Source: CAD feature listing. Evaluate the final solid. Frame: model axes, mm. Face numbers are marked on the shaded views. A direction names the side the tool comes from. Give positions to 0.01 mm unless a question says otherwise; leave off trailing zeros. Write each loop counter-clockwise with the first axis right and the second up, starting at its lowest first coordinate (ties: lowest second). Pieces come first, ordered by that corner, then holes. Notation, with made-up numbers: (-7.75, 63) -> (24.25, 63) arc R15 ccw to (24.25, 72) -> close; hole circle Ø1 at (75.25, 72). An arc over 180 degrees is marked (long way). Write item = value, one per line.
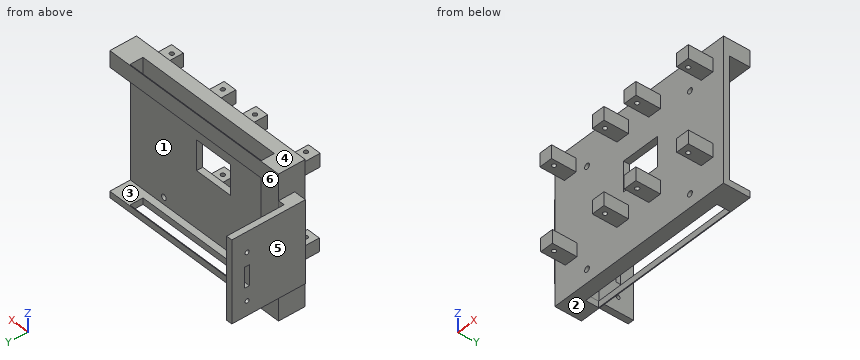
from build123d import *

# Parameters (mm, degrees)
SKETCH_1_W           = 95
SKETCH_1_H           = 70
SKETCH_1_R           = 1.35
SKETCH_1_W_2         = 19.026786566
SKETCH_1_H_2         = 14.673074928
EXTRUDE_1_DEPTH      = 13
SKETCH_3_W           = 85
SKETCH_3_H           = 59
CUT_EXTRUDE_1_DEPTH  = 10
SKETCH_4_W           = 6.551363844
SKETCH_4_H           = 6.551363844
EXTRUDE_2_DEPTH      = 12
SKETCH_7_W           = 6.551363844
SKETCH_7_H           = 6.551363844
EXTRUDE_3_DEPTH      = 12
SKETCH_9_R           = 1
CUT_EXTRUDE_4_DEPTH  = 63
SKETCH_5_R           = 1
CUT_EXTRUDE_5_DEPTH  = 56
SKETCH_12_W          = 6.551363844
SKETCH_12_H          = 6.551363844
EXTRUDE_4_DEPTH      = 12
SKETCH_13_R          = 1
CUT_EXTRUDE_6_DEPTH  = 9
SKETCH_15_R          = 1
CUT_EXTRUDE_7_DEPTH  = 51
SKETCH_17_W          = 6.551363844
SKETCH_17_H          = 6.551363844
EXTRUDE_5_DEPTH      = 12
SKETCH_18_R          = 1
CUT_EXTRUDE_8_DEPTH  = 12
SKETCH_19_R          = 1
CUT_EXTRUDE_9_DEPTH  = 12
SKETCH_20_W          = 40
SKETCH_20_H          = 7.86503053
EXTRUDE_6_DEPTH      = 6
SKETCH_21_W          = 2.903775518
SKETCH_21_H          = 40
EXTRUDE_7_DEPTH      = 28
SKETCH_22_W          = 74
SKETCH_22_H          = 6.331212291
CUT_EXTRUDE_10_DEPTH = 78
SKETCH_23_W          = 10
SKETCH_23_H          = 2.4
CUT_EXTRUDE_13_DEPTH = 10
SKETCH_25_R          = 1
CUT_EXTRUDE_14_DEPTH = 10


with BuildPart() as part:
    # 草图1 → 凸台-拉伸1 (new body)
    with BuildSketch(Plane(origin=(0, 0, 0), x_dir=(1, 0, 0), z_dir=(0, 1, 0))):
        with Locations((21.0257099, -17.142747506)):
            Rectangle(SKETCH_1_W, SKETCH_1_H)
        with Locations((49.670533911, 11.329362359)):
            Circle(SKETCH_1_R, mode=Mode.SUBTRACT)
        with Locations((49.670533911, -37.670637641)):
            Circle(SKETCH_1_R, mode=Mode.SUBTRACT)
        with Locations((-8.329466089, -37.670637641)):
            Circle(SKETCH_1_R, mode=Mode.SUBTRACT)
        with Locations((-8.329466089, 11.329362359)):
            Circle(SKETCH_1_R, mode=Mode.SUBTRACT)
        with Locations((21.72534394, -20.076013692)):
            Rectangle(SKETCH_1_W_2, SKETCH_1_H_2, mode=Mode.SUBTRACT)
    extrude(amount=EXTRUDE_1_DEPTH)

    # 草图3 → 切除-拉伸1 (cut)
    with BuildSketch(Plane(origin=(0, 13, 0), x_dir=(1, 0, 0), z_dir=(0, 1, 0))):
        with Locations((26.0257099, -14.722914633)):
            Rectangle(SKETCH_3_W, SKETCH_3_H)
    extrude(amount=-CUT_EXTRUDE_1_DEPTH, mode=Mode.SUBTRACT)

    # 草图4 → 凸台-拉伸2 (add)
    with BuildSketch(Plane.XZ):
        with Locations((-17.262018052, 1.397045451)):
            Rectangle(SKETCH_4_W, SKETCH_4_H)
        with Locations((-17.755298179, 42.036450596)):
            Rectangle(SKETCH_4_W, SKETCH_4_H)
        with Locations((59.313437853, 1.397045451)):
            Rectangle(SKETCH_4_W, SKETCH_4_H)
        with Locations((59.313437853, 42.036450596)):
            Rectangle(SKETCH_4_W, SKETCH_4_H)
    extrude(amount=EXTRUDE_2_DEPTH)

    # 草图7 → 凸台-拉伸3 (add)
    with BuildSketch(Plane.XZ):
        with Locations((29.762074009, 2.155967477)):
            Rectangle(SKETCH_7_W, SKETCH_7_H)
    extrude(amount=EXTRUDE_3_DEPTH)

    # 草图9 → 切除-拉伸4 (cut)
    with BuildSketch(Plane(origin=(0, 0, -1.119714445), x_dir=(-1, 0, 0), z_dir=(0, 0, -1))):
        with Locations((-29.819487591, -8.583293227)):
            Circle(SKETCH_9_R)
    extrude(amount=-CUT_EXTRUDE_4_DEPTH, mode=Mode.SUBTRACT)

    # 草图5 → 切除-拉伸5 (cut)
    with BuildSketch(Plane(origin=(0, 0, -1.878636471), x_dir=(-1, 0, 0), z_dir=(0, 0, -1))):
        with Locations((-58.566110561, -8.583293227)):
            Circle(SKETCH_5_R)
    extrude(amount=-CUT_EXTRUDE_5_DEPTH, mode=Mode.SUBTRACT)

    # 草图12 → 凸台-拉伸4 (add)
    with BuildSketch(Plane(origin=(0, 0, 0), x_dir=(-1, 0, 0), z_dir=(0, -1, 0))):
        with Locations((-29.762074009, -42.795372621)):
            Rectangle(SKETCH_12_W, SKETCH_12_H)
    extrude(amount=EXTRUDE_4_DEPTH)

    # 草图13 → 切除-拉伸6 (cut)
    with BuildSketch(Plane.XY.offset(46.071054543)):
        with Locations((29.819487591, -8.583293227)):
            Circle(SKETCH_13_R)
    extrude(amount=-CUT_EXTRUDE_6_DEPTH, mode=Mode.SUBTRACT)

    # 草图15 → 切除-拉伸7 (cut)
    with BuildSketch(Plane.XY.offset(45.312132518)):
        with Locations((-17.007970887, -8.583602404)):
            Circle(SKETCH_15_R)
    extrude(amount=-CUT_EXTRUDE_7_DEPTH, mode=Mode.SUBTRACT)

    # 草图17 → 凸台-拉伸5 (add)
    with BuildSketch(Plane(origin=(0, 0, 0), x_dir=(-1, 0, 0), z_dir=(0, -1, 0))):
        with Locations((-11.796065665, -42.036450596)):
            Rectangle(SKETCH_17_W, SKETCH_17_H)
        with Locations((-11.796065665, -1.397045451)):
            Rectangle(SKETCH_17_W, SKETCH_17_H)
    extrude(amount=EXTRUDE_5_DEPTH)

    # 草图18 → 切除-拉伸8 (cut)
    with BuildSketch(Plane.XY.offset(45.312132518)):
        with Locations((11.738652082, -8.583602404)):
            Circle(SKETCH_18_R)
    extrude(amount=-CUT_EXTRUDE_8_DEPTH, mode=Mode.SUBTRACT)

    # 草图19 → 切除-拉伸9 (cut)
    with BuildSketch(Plane(origin=(0, 0, -1.878636471), x_dir=(-1, 0, 0), z_dir=(0, 0, -1))):
        with Locations((-11.738652082, -8.583602404)):
            Circle(SKETCH_19_R)
    extrude(amount=-CUT_EXTRUDE_9_DEPTH, mode=Mode.SUBTRACT)

    # 草图20 → 凸台-拉伸6 (add)
    with BuildSketch(Plane.ZY.offset(26.4742901)):
        with Locations((19.434170465, 9.018379662)):
            Rectangle(SKETCH_20_W, SKETCH_20_H)
    extrude(amount=EXTRUDE_6_DEPTH)

    # 草图21 → 凸台-拉伸7 (add)
    with BuildSketch(Plane(origin=(0, 12.950894927, 0), x_dir=(1, 0, 0), z_dir=(0, 1, 0))):
        with Locations((-31.022402341, -19.434170465)):
            Rectangle(SKETCH_21_W, SKETCH_21_H)
    extrude(amount=EXTRUDE_7_DEPTH)

    # 草图22 → 切除-拉伸10 (cut)
    with BuildSketch(Plane(origin=(0, 0, -17.857252494), x_dir=(-1, 0, 0), z_dir=(0, 0, -1))):
        with Locations((-20.578648713, 9.467151169)):
            Rectangle(SKETCH_22_W, SKETCH_22_H)
    extrude(amount=-CUT_EXTRUDE_10_DEPTH, mode=Mode.SUBTRACT)

    # 草图23 → 切除-拉伸13 (cut)
    with BuildSketch(Plane.ZY.offset(32.4742901)):
        with Locations((18.096879679, 33.602818556)):
            Rectangle(SKETCH_23_W, SKETCH_23_H)
    extrude(amount=-CUT_EXTRUDE_13_DEPTH, mode=Mode.SUBTRACT)

    # 草图25 → 切除-拉伸14 (cut)
    with BuildSketch(Plane.ZY.offset(32.4742901)):
        with Locations((6.428608959, 33.489118381)):
            Circle(SKETCH_25_R)
        with Locations((29.528608959, 33.489118381)):
            Circle(SKETCH_25_R)
    extrude(amount=-CUT_EXTRUDE_14_DEPTH, mode=Mode.SUBTRACT)


solid = part.part
(1) First-contact query: pin 1 (6 mm diameter, centred on x = 26, z = -2.5, fed in from +Y); pin 2 (7 mm diameter, centred on y = 9, z = 46.5, fed in from -X); pin 3 (2 mm diameter, centred on y = -7, z = 43.5, fed in from -X); pin 4 (6 mm diameter, centred on x = -3.5, y = 6.5, fed in from +Z). Flat tips, straight axial feed; report the tip coordinate or a pass-through.
Values follow:
pin_1 = 3
pin_2 = -26.47
pin_3 = -21.03
pin_4 = 52.14
(2) Section query C-C (z = 25.5). Return loops of the section in (x, y), plus the area to 3 significant figures.
Values follow:
outline = (-32.47, 5.09) -> (-26.47, 5.09) -> (-26.47, 0) -> (12.21, 0) -> (12.21, 3) -> (-16.47, 3) -> (-16.47, 13) -> (-26.47, 13) -> (-26.47, 12.95) -> (-29.57, 12.95) -> (-29.57, 40.95) -> (-32.47, 40.95) -> close; (31.24, 0) -> (68.53, 0) -> (68.53, 3) -> (31.24, 3) -> close
area = 456 mm2
(3) Section query B-B (x = 53.5). Return loops of the section in (y, z).
Values follow:
outline = (0, -17.86) -> (6.3, -17.86) -> (6.3, -14.78) -> (3, -14.78) -> (3, 44.22) -> (6.3, 44.22) -> (6.3, 52.14) -> (0, 52.14) -> close; (12.63, -17.86) -> (13, -17.86) -> (13, -14.78) -> (12.63, -14.78) -> close; (12.63, 44.22) -> (13, 44.22) -> (13, 52.14) -> (12.63, 52.14) -> close
(4) Pull-direction query (Z, two-part tool) for the marked faces 1, 2, 3 and 4; classes: pulls with the +Z half, pulls with the -Z half, needs draft (parallel to the pull), parting line crosses it, or undercut.
Values follow:
face_1 = undercut
face_2 = pulls with the -Z half
face_3 = undercut
face_4 = pulls with the +Z half
(5) Section query D-D (y = 31). Return loops of the section in (x, z), plus the area to 3 significant figures.
Values follow:
outline = (-32.47, -0.57) -> (-29.57, -0.57) -> (-29.57, 39.43) -> (-32.47, 39.43) -> close
area = 116 mm2
(6) Material intervals for line 1 (Z direction, x = 60.5, y = 7.5); line 2 (X direction, y = -8.5, z = 46); line 3 (Y direction, x = -3.5, z = -3.5), sorted ascending.
Values follow:
line_1 = -17.86 to -14.78, 44.22 to 52.14
line_2 = 26.49 to 28.82, 30.82 to 33.04
line_3 = 0 to 3
(7) Access query for the marked faces 5 and 6. Directions: +Z, -Z, +X, -X, +Y, -Y. A direction counts if a zero-diameter tool reaches every point of the face in a straight line with its end or side. Return the directions, or none.
Values follow:
face_5 = +Z, -Z, -X, +Y, -Y
face_6 = +Z, -Z, +X, +Y
(8) Section query A-A (z = 17). Return loops of the section in (x, y).
Values follow:
outline = (-32.47, 5.09) -> (-26.47, 5.09) -> (-26.47, 0) -> (12.21, 0) -> (12.21, 3) -> (-16.47, 3) -> (-16.47, 13) -> (-26.47, 13) -> (-26.47, 12.95) -> (-29.57, 12.95) -> (-29.57, 32.4) -> (-32.47, 32.4) -> close; (-32.47, 34.8) -> (-29.57, 34.8) -> (-29.57, 40.95) -> (-32.47, 40.95) -> close; (31.24, 0) -> (68.53, 0) -> (68.53, 3) -> (31.24, 3) -> close
